Part model, mm, in its own coordinate system. Face numbers are marked on the shaded views. A direction names the side the tool comes from. Round coordinates to 2 decimals unless told otherwise and drop trailing zeros. Loops run counter-clockwise (first coordinate to the right, second up) from the corner with the lowest first, then second, coordinate; pieces in that order, holes last.
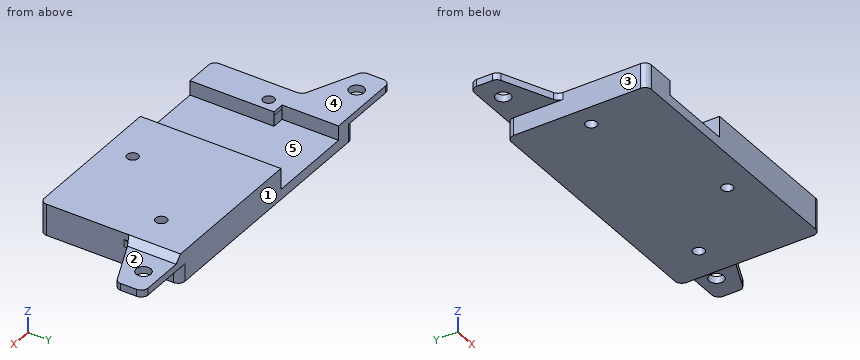
from build123d import *

# Parameters (mm, degrees)
BOSS_EXTRUDE1_DEPTH  = 5.1
SKETCH2_R            = 2.1
BOSS_EXTRUDE2_DEPTH  = 0.9
FILLET1_R            = 2
SKETCH3_R            = 2.1
BOSS_EXTRUDE3_DEPTH  = 1.1
BOSS_EXTRUDE4_DEPTH  = 16.158031
SKETCH5_W            = 25
SKETCH5_H            = 40.2
CUT_EXTRUDE2_DEPTH   = 3.05
SKETCH6_W            = 6
SKETCH6_H            = 24.2
BOSS_EXTRUDE5_DEPTH  = 3.5
CUT_EXTRUDE3_DEPTH   = 16.158031
BOSS_EXTRUDE6_DEPTH  = 3
BOSS_EXTRUDE7_REACH  = 42.2
SKETCH21_R           = 1.6
CUT_EXTRUDE6_DEPTH   = 9
CUT_EXTRUDE7_DEPTH   = 17.15803115
SKETCH23_W           = 1.1
SKETCH23_H           = 16.15803115
BOSS_EXTRUDE9_DEPTH  = 6.39
SKETCH26_W           = 3.5
SKETCH26_H           = 3.05
CUT_EXTRUDE11_DEPTH  = 0.158031
BOSS_EXTRUDE10_DEPTH = 1.1
SKETCH28_R           = 1.6
CUT_EXTRUDE12_DEPTH  = 7.1


with BuildPart() as part:
    # Sketch1 → Boss-Extrude1 (new body)
    with BuildSketch(Plane.XY):
        with BuildLine():
            Line((99.95, 149.85), (25.05, 149.85))
            Line((25.05, 149.85), (25.05, 148))
            Line((25.05, 148), (25.05, 111.5))
            ThreePointArc((25.05, 111.5), (25.591852455, 110.191852455), (26.9, 109.65))
            Line((26.9, 109.65), (98.1, 109.65))
            ThreePointArc((98.1, 109.65), (99.408147545, 110.191852455), (99.95, 111.5))
            Line((99.95, 111.5), (99.95, 148))
            Line((99.95, 148), (99.95, 149.85))
        make_face()
    extrude(amount=BOSS_EXTRUDE1_DEPTH)

    # Sketch2 → Boss-Extrude2 (add)
    with BuildSketch(Plane.XY.offset(5.1)):
        with BuildLine():
            Line((102.1, 149.85), (22.9, 149.85))
            Line((22.9, 149.85), (9.05, 149.85))
            Line((9.05, 149.85), (9.05, 148))
            Line((9.05, 148), (9.05, 143.30803115))
            ThreePointArc((9.05, 143.30803115), (9.351726371, 142.295436082), (10.158485157, 141.61314008))
            Line((10.158485157, 141.61314008), (23.761760493, 135.66170712))
            ThreePointArc((23.761760493, 135.66170712), (24.699345028, 134.868768523), (25.05, 133.69196885))
            Line((25.05, 133.69196885), (25.05, 111.5))
            ThreePointArc((25.05, 111.5), (25.591852455, 110.191852455), (26.9, 109.65))
            Line((26.9, 109.65), (98.1, 109.65))
            ThreePointArc((98.1, 109.65), (99.408147545, 110.191852455), (99.95, 111.5))
            Line((99.95, 111.5), (99.95, 133.69196885))
            ThreePointArc((99.95, 133.69196885), (100.300654972, 134.868768523), (101.238239507, 135.66170712))
            Line((101.238239507, 135.66170712), (114.841514843, 141.61314008))
            ThreePointArc((114.841514843, 141.61314008), (115.648273629, 142.295436082), (115.95, 143.30803115))
            Line((115.95, 143.30803115), (115.95, 148))
            Line((115.95, 148), (115.95, 149.85))
            Line((115.95, 149.85), (102.1, 149.85))
        make_face()
        with Locations((16.3, 145.05)):
            Circle(SKETCH2_R, mode=Mode.SUBTRACT)
        with Locations((108.7, 145.05)):
            Circle(SKETCH2_R, mode=Mode.SUBTRACT)
    extrude(amount=BOSS_EXTRUDE2_DEPTH)

    # Fillet1
    fillet1_edges = [part.edges().sort_by_distance(p)[0] for p in [
        (25.05, 149.85, 2.55),
        (99.95, 149.85, 2.55),
        (115.95, 149.85, 5.55),
        (9.05, 149.85, 5.55),
    ]]
    fillet(fillet1_edges, radius=FILLET1_R)

    # Sketch3 → Boss-Extrude3 (add)
    with BuildSketch(Plane.XY.offset(6)):
        with BuildLine():
            Line((99.95, 133.69196885), (99.95, 149.85))
            Line((99.95, 149.85), (113.95, 149.85))
            ThreePointArc((113.95, 149.85), (115.364213562, 149.264213562), (115.95, 147.85))
            Line((115.95, 147.85), (115.95, 143.30803115))
            ThreePointArc((115.95, 143.30803115), (115.648273629, 142.295436082), (114.841514843, 141.61314008))
            Line((114.841514843, 141.61314008), (101.238239507, 135.66170712))
            ThreePointArc((101.238239507, 135.66170712), (100.300654972, 134.868768523), (99.95, 133.69196885))
        make_face()
        with Locations((108.7, 145.05)):
            Circle(SKETCH3_R, mode=Mode.SUBTRACT)
        with BuildLine():
            Line((11.05, 149.85), (25.05, 149.85))
            Line((25.05, 149.85), (25.05, 133.69196885))
            ThreePointArc((25.05, 133.69196885), (24.699345028, 134.868768523), (23.761760493, 135.66170712))
            Line((23.761760493, 135.66170712), (10.158485157, 141.61314008))
            ThreePointArc((10.158485157, 141.61314008), (9.351726371, 142.295436082), (9.05, 143.30803115))
            Line((9.05, 143.30803115), (9.05, 147.85))
            ThreePointArc((9.05, 147.85), (9.635786438, 149.264213562), (11.05, 149.85))
        make_face()
        with Locations((16.3, 145.05)):
            Circle(SKETCH3_R, mode=Mode.SUBTRACT)
    extrude(amount=BOSS_EXTRUDE3_DEPTH)

    # Sketch4 → Boss-Extrude4 (add)
    with BuildSketch(Plane(origin=(0, 149.85, 0), x_dir=(1, 0, 0), z_dir=(0, 1, 0))):
        Polygon((25.05, -7.1), (27.55, -6), (25.05, -6), align=None)
        Polygon((97.45, -6), (99.95, -7.1), (99.95, -6), align=None)
    extrude(amount=-BOSS_EXTRUDE4_DEPTH)

    # Sketch5 → Cut-Extrude2 (cut)
    with BuildSketch(Plane.XY.offset(6)):
        with Locations((43.94, 129.75)):
            Rectangle(SKETCH5_W, SKETCH5_H)
    extrude(amount=-CUT_EXTRUDE2_DEPTH, mode=Mode.SUBTRACT)

    # Sketch6 → Boss-Extrude5 (add)
    with BuildSketch(Plane(origin=(31.44, 0, 0), x_dir=(0, 0, -1), z_dir=(1, 0, 0))):
        with Locations((-3, 121.75)):
            Rectangle(SKETCH6_W, SKETCH6_H)
    extrude(amount=BOSS_EXTRUDE5_DEPTH)

    # Sketch9 → Cut-Extrude3 (cut)
    with BuildSketch(Plane.XZ.offset(-133.69196885)):
        Polygon((97.45, 6), (99.95, 7.1), (99.95, 6), align=None)
    extrude(amount=-CUT_EXTRUDE3_DEPTH, mode=Mode.SUBTRACT)

    # Sketch10 → Boss-Extrude6 (add)
    with BuildSketch(Plane.XY.offset(6)):
        with BuildLine():
            Line((56.44, 149.85), (56.44, 109.65))
            Line((56.44, 109.65), (98.1, 109.65))
            ThreePointArc((98.1, 109.65), (99.408147545, 110.191852455), (99.95, 111.5))
            Line((99.95, 111.5), (99.95, 149.85))
            Line((99.95, 149.85), (56.44, 149.85))
        make_face()
    extrude(amount=BOSS_EXTRUDE6_DEPTH)

    # Boss-Extrude7: up to this face of the body (flat: up to its plane)
    boss_extrude7_end = Plane(part.part.faces().sort_by_distance((108.039877175, 138.6374236, 6.1))[0])
    # Sketch12 → Boss-Extrude7 (add, up to the picked face)
    with BuildSketch(Plane(origin=(0, 149.85, 0), x_dir=(1, 0, 0), z_dir=(0, 1, 0)), mode=Mode.PRIVATE) as boss_extrude7_sk1:
        Polygon((99.95, -9), (99.95, -7.1), (101.85, -7.1), align=None)
    boss_extrude7_tool1 = split(extrude(boss_extrude7_sk1.sketch, amount=-BOSS_EXTRUDE7_REACH, mode=Mode.PRIVATE), bisect_by=boss_extrude7_end, keep=Keep.BOTH, mode=Mode.PRIVATE)
    add(boss_extrude7_tool1.solids().sort_by_distance((100.583333, 149.85, 7.733333))[0])

    # Sketch21 → Cut-Extrude6 (cut)
    with BuildSketch(Plane.XY.offset(9)):
        with Locations((90.44, 138.06)):
            Circle(SKETCH21_R)
        with Locations((71.69, 117.51)):
            Circle(SKETCH21_R)
    extrude(amount=-CUT_EXTRUDE6_DEPTH, mode=Mode.SUBTRACT)

    # Sketch22 → Cut-Extrude7 (cut, through all)
    with BuildSketch(Plane.XZ.offset(-133.69196885)):
        Polygon((25.05, 7.1), (25.05, 6), (27.55, 6), align=None)
    extrude(amount=-CUT_EXTRUDE7_DEPTH, mode=Mode.SUBTRACT)

    # Sketch23 → Boss-Extrude9 (add)
    with BuildSketch(Plane(origin=(25.05, 0, 0), x_dir=(0, 0, -1), z_dir=(1, 0, 0))):
        with Locations((-6.55, 141.770984425)):
            Rectangle(SKETCH23_W, SKETCH23_H)
    extrude(amount=BOSS_EXTRUDE9_DEPTH)

    # Sketch26 → Cut-Extrude11 (cut)
    with BuildSketch(Plane(origin=(0, 133.85, 0), x_dir=(1, 0, 0), z_dir=(0, 1, 0))):
        with Locations((33.19, -4.475)):
            Rectangle(SKETCH26_W, SKETCH26_H)
    extrude(amount=-CUT_EXTRUDE11_DEPTH, mode=Mode.SUBTRACT)

    # Sketch27 → Boss-Extrude10 (add)
    with BuildSketch(Plane.XY.offset(6)):
        with BuildLine():
            Line((34.94, 109.65), (34.94, 133.69196885))
            Line((34.94, 133.69196885), (25.05, 133.69196885))
            Line((25.05, 133.69196885), (25.05, 111.5))
            ThreePointArc((25.05, 111.5), (25.591852455, 110.191852455), (26.9, 109.65))
            Line((26.9, 109.65), (34.94, 109.65))
        make_face()
    extrude(amount=BOSS_EXTRUDE10_DEPTH)

    # Sketch28 → Cut-Extrude12 (cut)
    with BuildSketch(Plane.XY.offset(7.1)):
        with Locations((31.295, 129.75)):
            Circle(SKETCH28_R)
    extrude(amount=-CUT_EXTRUDE12_DEPTH, mode=Mode.SUBTRACT)


solid = part.part
1) Wall check: line 1 along X through (y, z) = (145.05, 5.75); line 2 along X through (y, z) = (138.06, 3.75); line 3 along X through (y, z) = (128, 5). Give the ranges that are in metal, low to high.
Values:
line 1: x = 9.05 to 14.2, 18.4 to 31.44, 56.44 to 106.6, 110.8 to 115.95
line 2: x = 25.05 to 31.44, 56.44 to 88.84, 92.04 to 99.95
line 3: x = 25.05 to 34.94, 56.44 to 99.95
2) Slice it at B-B, the plane x = 71.69. Give the cut face in (y, z).
Values:
outline: (109.65, 0) - (115.91, 0) - (115.91, 9) - (109.65, 9) - close; (119.11, 0) - (149.85, 0) - (149.85, 9) - (119.11, 9) - close
3) Tool access for the marked faces 1 and 2: list every direction of +Z, -Z, +X, -X, +Y, -Y with a clear straight run to the whole face (end or side of a thin tool).
Values:
face 1: +Z, -Z, +X, -X, +Y
face 2: +Z, +X, +Y, -Y
4) Slice it at A-A, the plane y = 129.75. Give the cut face in (x, z) (3 decimals), then the cut area to 3 significant figures.
Values:
outline: (25.05, 0) - (29.695, 0) - (29.695, 7.1) - (25.05, 7.1) - close; (32.895, 0) - (99.95, 0) - (99.95, 9) - (56.44, 9) - (56.44, 2.95) - (34.94, 2.95) - (34.94, 7.1) - (32.895, 7.1) - close
area: 503 mm2
5) Slice it at D-D, the plane z = 1.75. Give the cut face in (x, y) (3 decimals), then the cut area to 3 significant figures.
Values:
outline: (25.05, 111.5) arc R1.85 ccw to (26.9, 109.65) - (98.1, 109.65) arc R1.85 ccw to (99.95, 111.5) - (99.95, 147.85) arc R2 ccw to (97.95, 149.85) - (27.05, 149.85) arc R2 ccw to (25.05, 147.85) - close; hole circle Ø3.2 at (31.295, 129.75); hole circle Ø3.2 at (71.69, 117.51); hole circle Ø3.2 at (90.44, 138.06)
area: 2,980 mm2
6) Mould opens along X. For the marked faces 3, 4 and 5 say: released by +X, released by -X, zero draft, split by the parting line, or undercut.
Values:
face 3: released by -X
face 4: zero draft
face 5: undercut
7) Slice it at C-C, the plane y = 145.05. Give the cut face in (x, z), then the cut area to 3 significant figures.
Values:
outline: (9.05, 5.1) - (14.2, 5.1) - (14.2, 7.1) - (9.05, 7.1) - close; (18.4, 5.1) - (25.05, 5.1) - (25.05, 0) - (99.95, 0) - (99.95, 5.1) - (106.6, 5.1) - (106.6, 7.1) - (101.85, 7.1) - (99.95, 9) - (56.44, 9) - (56.44, 2.95) - (31.44, 2.95) - (31.44, 7.1) - (18.4, 7.1) - close; (110.8, 5.1) - (115.95, 5.1) - (115.95, 7.1) - (110.8, 7.1) - close
area: 560 mm2
8) Drop flat-ended pins along their axis: pin 1 Ø2.5 at (y, z) = (128.5, 5.5) entering from +X; pin 2 Ø5 at (x, y) = (16.3, 145.05) entering from -Z; pin 3 Ø12.5 at (x, y) = (49, 129) entering from +Z; pin 4 Ø3 at (x, y) = (71.69, 117.51) entering from +Z. Give the stop position or say it passes through.
Values:
pin 1: stops at x = 99.95
pin 2: stops at z = 5.1
pin 3: stops at z = 2.95
pin 4: passes through
